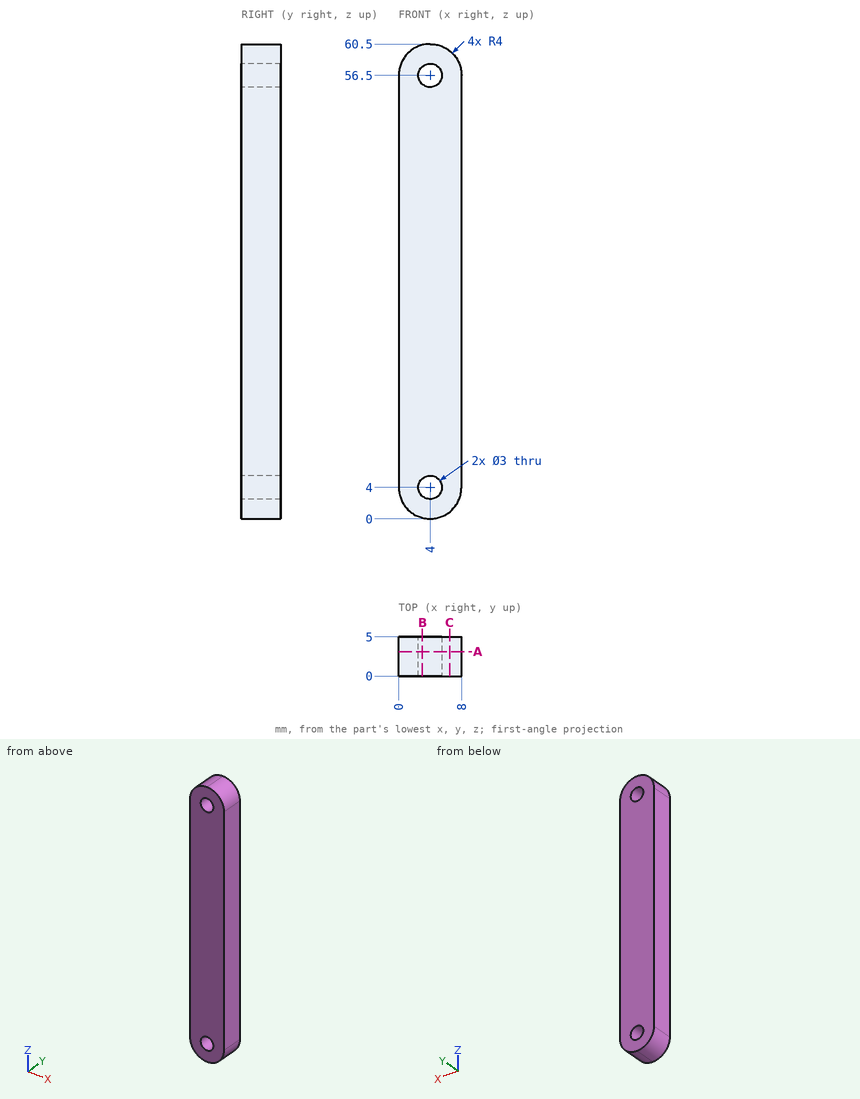
Can you work these out from the drawing? Everything is in mm from the part's minimum corner. Give positions to 0.01 mm unless a question says otherwise; leave off trailing zeros. Order: outer loops, then holes, each group sorted by start corner. A loop starts at its lowest first (then second) coordinate and runs counter-clockwise, first axis right, second up. Notation, with made-up numbers: M 56,43.25 L 107,43.25 A10 ccw 107,56.25 Z; hole C 52,-31 d2. An arc over 180 degrees is marked long. Write item = value, one per line. Start each with the question number.
Q1. Suppose I cut it at A-A (y = 3.1). Count the separate pieces of the cut face and the enclosed holes in it, plus the area to 3 significant figures.
Q2. Suppose I cut it at C-C (x = 6.5). Write out the boundary of the cut face in (y, z), plus the area to 3 significant figures.
Q3. Suppose I cut it at B-B (x = 3). Write out the boundary of the cut face in (y, z).
Q4. Will these pins go through, and if not, where does the flat tip stop? pin 1 Ø2.5 at (x, z) = (4, 4) entering from +Y; pin 2 Ø3 at (x, y) = (7, 0.5) entering from -Z.
Q5. I need wall thicknesses on probe 1 along Z at (x, y) = (4, 2.9); probe 2 along Z at (x, y) = (3.5, 2.5); probe 3 along X at (y, z) = (1.95, 55.5). Which ranges of each line are inside material? Lowest first, please. Write a range as [from, to].
Check result:
q1.separate_pieces = 1
q1.enclosed_holes = 2
q1.area = 456 mm2
q2.outline = M 0,0.88 L 5,0.88 L 5,59.62 L 0,59.62 Z
q2.area = 294 mm2
q3.outline = M 0,0.13 L 5,0.13 L 5,2.88 L 0,2.88 Z; M 0,5.12 L 5,5.12 L 5,55.38 L 0,55.38 Z; M 0,57.62 L 5,57.62 L 5,60.37 L 0,60.37 Z
q4.pin_1 = through
q4.pin_2 = 0.29
q5.probe_1 = [0, 2.5], [5.5, 55], [58, 60.5]
q5.probe_2 = [0.03, 2.59], [5.41, 55.09], [57.91, 60.47]
q5.probe_3 = [0, 2.88], [5.12, 8]
